Model file for the job. Use its own axes, mm. Face numbers are marked on the shaded views. A direction names the side the tool comes from. Give positions to 0.01 mm unless a question says otherwise; leave off trailing zeros. Order: outer loops, then holes, each group sorted by start corner. A loop starts at its lowest first (then second) coordinate and runs counter-clockwise, first axis right, second up. Notation, with made-up numbers: (-29, 88.25) - (24, 88.25) arc R20 cw to (24, 113.25) - close; hole circle Ø9 at (4, 25.5). An arc over 180 degrees is marked (long way). Use CSV: the item, a comma, the result in double quotes. Start each with the question number.
(1) Probe L1, parallel to X at y = 2.75, z = -7.5; L2, parallel to Z at x = -0.5, y = 1.25; L3, parallel to X at y = 3.3, z = -6. List the from-to ranges inside material, lowest first.
(2) Band-saw the part on A-A, the plane x = 0. Give the cut face in (y, z), then the cut area to 3 significant figures.
(3) Drop flat-ended pins along their axis: pin 1 Ø4 at (x, z) = (-5, -12.5) entering from -Y; pin 2 Ø0.9 at (y, z) = (3.5, -5) entering from +X; pin 3 Ø2 at (y, z) = (3.5, -13.5) entering from -X; pin 4 Ø0.9 at (y, z) = (2, -5.5) entering from -X. Give the stop position or say it passes through.
(4) Pull direction X, two halves, no side cores. Call the marked faces 3, 4 and 5: +X half, -X half, draft (parallel to the pull), parting line (faces both ways), or undercut.
(5) Tool access for the marked faces 1 and 2: list every direction of +Z, -Z, +X, -X, +Y, -Y with a clear straight run to the whole face (end or side of a thin tool).
(6) Band-saw the part on D-D, the plane z = -13.75. Give the cut face in (x, y), then the cut area to 3 significant figures.
(7) Band-saw the part on B-B, the plane y = 3.4. Give the cut face in (x, z), then the cut area to 3 significant figures.
(8) Band-saw the part on C-C, the plane z = -3. Give the cut face in (x, y).
from build123d import *

# Parameters (mm, degrees)
BOSS_EXTRUDE1_DEPTH = 5.0038


with BuildPart() as part:
    # Sketch1 → Boss-Extrude1 (new body)
    with BuildSketch(Plane(origin=(0, 0, 0), x_dir=(1, 0, 0), z_dir=(0, 1, 0))):
        Polygon((-8.9027, 0), (8.9027, 0), (8.9027, 3.81), (4.8514, 15.24), (-4.8514, 15.24), (-8.9027, 3.81), align=None)
        with BuildLine():
            Line((-1.4986, 3.81), (-1.4986, 6.8072))
            ThreePointArc((-1.4986, 6.8072), (0, 8.3058), (1.4986, 6.8072))
            Line((1.4986, 6.8072), (1.4986, 3.81))
            ThreePointArc((1.4986, 3.81), (0, 2.3114), (-1.4986, 3.81))
        make_face(mode=Mode.SUBTRACT)
    extrude(amount=BOSS_EXTRUDE1_DEPTH)


solid = part.part
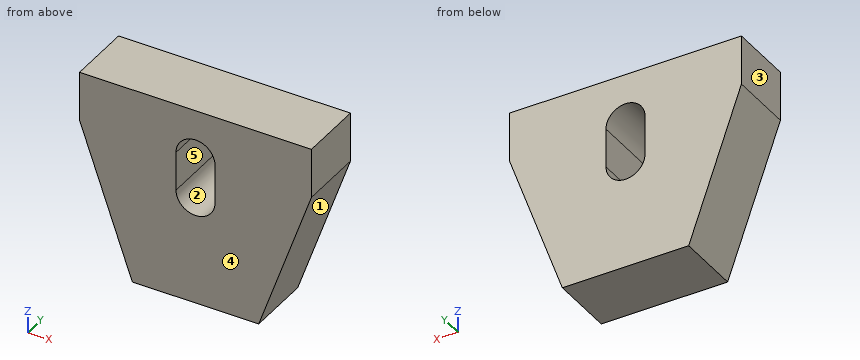
Answer block:
1,L1,"x = -7.59 to -1.33, 1.33 to 7.59"
1,L2,"z = -15.24 to -8.22, -2.4 to 0"
1,L3,"x = -8.13 to -1.5, 1.5 to 8.13"
2,outline,"(0, -15.24) - (5, -15.24) - (5, -8.31) - (0, -8.31) - close; (0, -2.31) - (5, -2.31) - (5, 0) - (0, 0) - close"
2,area,"46.3 mm2"
3,pin 1,"stops at y = 0"
3,pin 2,"stops at x = 8.64"
3,pin 3,"stops at x = -5.82"
3,pin 4,"stops at x = -8.46"
4,face 3,"-X half"
4,face 4,"draft"
4,face 5,"undercut"
5,face 1,"-Z, +X, +Y, -Y"
5,face 2,"+Y, -Y"
6,outline,"(-5.38, 0) - (5.38, 0) - (5.38, 5) - (-5.38, 5) - close"
6,area,"53.8 mm2"
7,outline,"(-8.9, -3.81) - (-4.85, -15.24) - (4.85, -15.24) - (8.9, -3.81) - (8.9, 0) - (-8.9, 0) - close; hole (-1.5, -6.81) arc R1.5 ccw to (1.5, -6.81) - (1.5, -3.81) arc R1.5 ccw to (-1.5, -3.81) - close"
7,area,"209 mm2"
8,outline,"(-8.9, 0) - (-1.26, 0) - (-1.26, 5) - (-8.9, 5) - close; (1.26, 0) - (8.9, 0) - (8.9, 5) - (1.26, 5) - close"
